Answer from the drawing. Dimensions are ordinates in mm from the lowest x, y and z of the part. Coordinates: 2 decimals unless noted, no trailing zeros. Write each loop counter-clockwise with the first axis right and the second up, starting at its lowest first coordinate (ties: lowest second). Pieces come first, ordered by that corner, then holes.
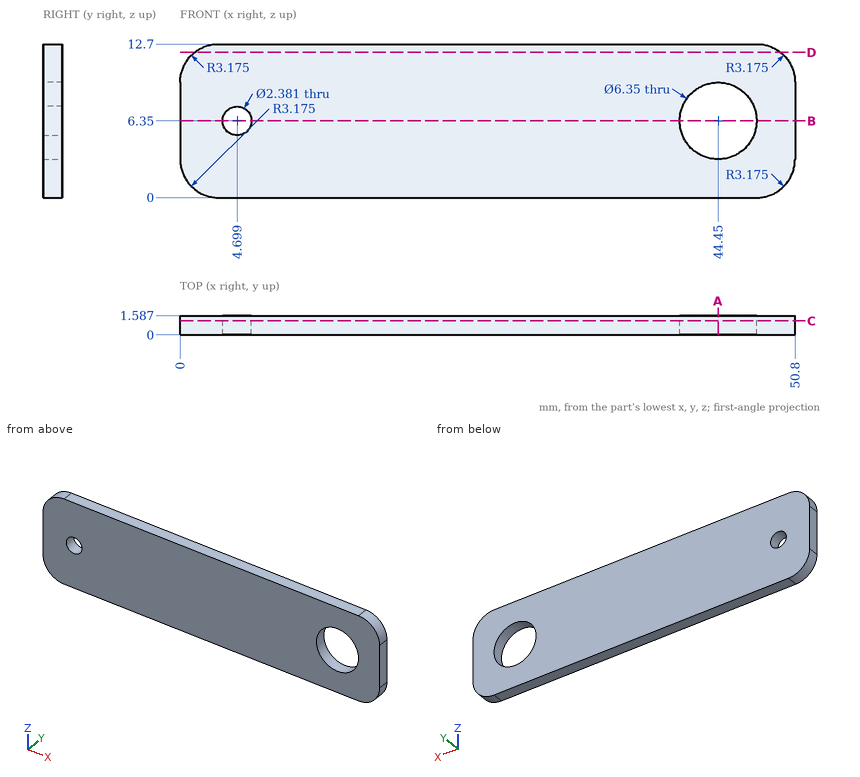
(1) Section C-C, the plane y = 1.15 is taken. State how many separate pieces and enclosed holes the cut face has.
(2) Section B-B, the plane z = 6.35 is taken. Write down the section's boundary in (x, y) (1 decimal).
(3) Find the intervals of material crossed by probe 1 along X at (y, z) = (1, 6.35) (1 decimal); probe 2 along X at (y, z) = (1, 7) (1 decimal); probe 3 along X at (y, z) = (0.45, 3.75) (1 decimal), in increasing order.
(4) Section A-A, the plane x = 44.45 is taken. Write down the section's boundary in (y, z) (1 decimal), plus the area to 3 significant figures.
(5) Section D-D, the plane z = 12 is taken. Write down the section's boundary in (x, y).
Solution:
1. separate pieces: 1
1. enclosed holes: 2
2. outline: (0, 0) - (3.5, 0) - (3.5, 1.6) - (0, 1.6) - close; (5.9, 0) - (41.3, 0) - (41.3, 1.6) - (5.9, 1.6) - close; (47.6, 0) - (50.8, 0) - (50.8, 1.6) - (47.6, 1.6) - close
3. probe 1: x = 0 to 3.5, 5.9 to 41.3, 47.6 to 50.8
3. probe 2: x = 0 to 3.7, 5.7 to 41.3, 47.6 to 50.8
3. probe 3: x = 0 to 42.6, 46.3 to 50.8
4. outline: (0, 0) - (1.6, 0) - (1.6, 3.2) - (0, 3.2) - close; (0, 9.5) - (1.6, 9.5) - (1.6, 12.7) - (0, 12.7) - close
4. area: 10.1 mm2
5. outline: (1.19, 0) - (49.61, 0) - (49.61, 1.59) - (1.19, 1.59) - close
